```python
from build123d import *

# Parameters (mm, degrees)
SKETCH1_W           = 104
SKETCH1_H           = 83.5
BOSS_EXTRUDE1_DEPTH = 55
SKETCH2_W           = 59.042208754
SKETCH2_H           = 15
CUT_EXTRUDE1_DEPTH  = 145.267979815
SKETCH3_R           = 1.5
CUT_EXTRUDE2_DEPTH  = 145.267979815
SKETCH4_W           = 40
SKETCH4_H           = 40
BOSS_EXTRUDE2_DEPTH = 10.5


with BuildPart() as part:
    # Sketch1 → Boss-Extrude1 (new body)
    with BuildSketch(Plane(origin=(0, 0, 0), x_dir=(1, 0, 0), z_dir=(0, 1, 0))):
        with Locations((52, 41.75)):
            Rectangle(SKETCH1_W, SKETCH1_H)
    extrude(amount=BOSS_EXTRUDE1_DEPTH)

    # Sketch2 → Cut-Extrude1 (cut, through all)
    with BuildSketch(Plane(origin=(104, 0, 0), x_dir=(0, 0, -1), z_dir=(1, 0, 0))):
        with Locations((53.978895623, 47.5)):
            Rectangle(SKETCH2_W, SKETCH2_H)
    extrude(amount=-CUT_EXTRUDE1_DEPTH, mode=Mode.SUBTRACT)

    # Sketch3 → Cut-Extrude2 (cut, through all)
    with BuildSketch(Plane.XZ):
        with Locations(Location((3.5, -79.75, 0), (0, 0, 270))):
            Circle(SKETCH3_R)
        with Locations(Location((3.5, -3.75, 0), (0, 0, 270))):
            Circle(SKETCH3_R)
        with Locations(Location((100.5, -3.75, 0), (0, 0, 270))):
            Circle(SKETCH3_R)
        with Locations(Location((100.5, -79.75, 0), (0, 0, 270))):
            Circle(SKETCH3_R)
    extrude(amount=-CUT_EXTRUDE2_DEPTH, mode=Mode.SUBTRACT)

    # Sketch4 → Boss-Extrude2 (add)
    with BuildSketch(Plane.ZY):
        with Locations((-26.35, 28)):
            Rectangle(SKETCH4_W, SKETCH4_H)
    extrude(amount=BOSS_EXTRUDE2_DEPTH)


solid = part.part
```
Could you check a few things on this model? Use its own coordinates, in mm. A direction names the side the tool comes from. Round coordinates to 2 decimals unless told otherwise and drop trailing zeros. Loops run counter-clockwise (first coordinate to the right, second up) from the corner with the lowest first, then second, coordinate; pieces in that order, holes last. Notation, with made-up numbers: (79.25, 87.25) - (104.25, 87.25) arc R19 ccw to (104.25, 109.25) - close; hole circle Ø1 at (54, 60.5). An arc over 180 degrees is marked (long way). Use CSV: the item, a comma, the result in double quotes.
Item 1: If we section it at D-D on z = -19.5: List the corners of the cut face in (x, y) for me.
Here are the results:
outline,"(-10.5, 8) - (0, 8) - (0, 0) - (104, 0) - (104, 55) - (0, 55) - (0, 48) - (-10.5, 48) - close"
Item 2: If we mould it in two halves opening along X, with no side actions, what happens to faces 1 (the flat face through (-10.5, 28, -27)), 2 (the cylindrical face through (2.925, 27.115, -5.136)), 3 (the flat face through (51, 20, -83.5))? For each: pulls with the +X half, pulls with the -X half, needs draft (parallel to the pull), parting line crosses it, or undercut.
Here are the results:
face 1,"pulls with the -X half"
face 2,"undercut"
face 3,"needs draft"
Item 3: If we section it at B-B on x = 100.5: List the corners of the cut face in (y, z) for me, then the cut area to 3 significant figures.
Here are the results:
outline,"(0, -83.5) - (40, -83.5) - (40, -81.25) - (0, -81.25) - close; (0, -78.25) - (40, -78.25) - (40, -24.46) - (55, -24.46) - (55, -5.25) - (0, -5.25) - close; (0, -2.25) - (55, -2.25) - (55, 0) - (0, 0) - close"
area,"3,420 mm²"
Item 4: For faces 4 (the flat face through (-5, 48, -27)), 5 (the flat face through (-5, 8, -27)), 6 (the flat face through (-5, 28, -6.35)), 7 (the flat face through (-5, 28, -46.35)), which set-ups out of +Z, -Z, +X, -X, +Y, -Y let a thin tool reach every point of the face, with its end or its side?
Here are the results:
face 4,"+Z, -Z, -X, +Y"
face 5,"+Z, -Z, -X, -Y"
face 6,"+Z, -X, +Y, -Y"
face 7,"-Z, -X, +Y, -Y"
Item 5: I need wall thicknesses on L1, parallel to Z at x = 100.5, y = 31; L2, parallel to X at y = 20, z = -79.75; L3, parallel to Z at x = 100.5, y = 43. Which ranges of each line are inside material? Lowest first, please. Write a range as [from, to].
Here are the results:
L1,"z = [-83.5, -81.25], [-78.25, -5.25], [-2.25, 0]"
L2,"x = [0, 2], [5, 99], [102, 104]"
L3,"z = [-24.46, -5.25], [-2.25, 0]"
Item 6: Will these pins go through, and if not, where does the flat tip stop? pin 1 (5 mm diameter, centred on x = 100.5, z = -79.75, fed in from -Y); pin 2 (5 mm diameter, centred on x = -8, z = -33, fed in from +Y); pin 3 (8 mm diameter, centred on x = 22.5, z = -47.5, fed in from +Y); pin 4 (4 mm diameter, centred on y = 44, z = -34, fed in from +X).
Here are the results:
pin 1,"stops at y = 0"
pin 2,"stops at y = 48"
pin 3,"stops at y = 40"
pin 4,"stops at x = 0"
Item 7: If we section it at A-A on z = -79.75: List the corners of the cut face in (x, y) for me, then the cut area to 3 significant figures.
Here are the results:
outline,"(0, 0) - (2, 0) - (2, 40) - (0, 40) - close; (5, 0) - (99, 0) - (99, 40) - (5, 40) - close; (102, 0) - (104, 0) - (104, 40) - (102, 40) - close"
area,"3,920 mm²"
Item 8: If we section it at C-C on y = 32: List the corners of the cut face in (x, z) for me, then the cut area to 3 significant figures.
Here are the results:
outline,"(-10.5, -46.35) - (0, -46.35) - (0, -83.5) - (104, -83.5) - (104, 0) - (0, 0) - (0, -6.35) - (-10.5, -6.35) - close; hole circle Ø3 at (3.5, -79.75); hole circle Ø3 at (3.5, -3.75); hole circle Ø3 at (100.5, -79.75); hole circle Ø3 at (100.5, -3.75)"
area,"9,080 mm²"
